Input: part model. Units: mm. Frame: model coordinates. Face numbers are marked on the shaded views. A direction names the side the tool comes from. Give positions to 0.01 mm unless a question says otherwise; leave off trailing zeros. Loops run counter-clockwise (first coordinate to the right, second up) from the corner with the lowest first, then second, coordinate; pieces in that order, holes last. Notation, with made-up numbers: M 76,84 L 116,84 A30 cw 116,123 Z; hole C 46.25,1 d9. An arc over 180 degrees is marked long. Return JSON: item names as keys, results as strings. Group by question number.
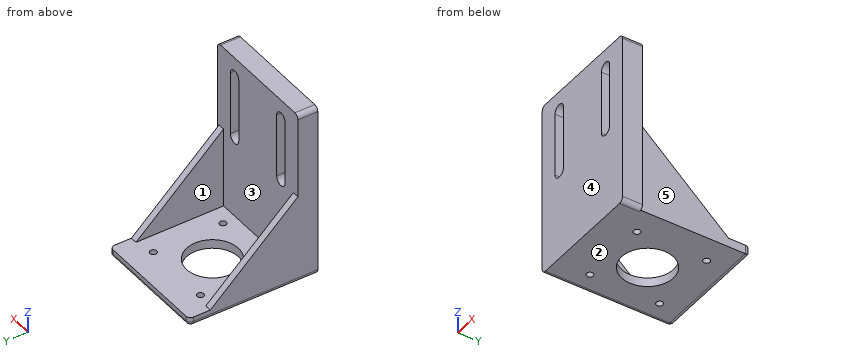
```python
from build123d import *

# Parameters (mm, degrees)
SKETCH1_W               = 53
SKETCH1_H               = 78
BOSS_EXTRUDE1_DEPTH     = 8.85
FILLET2_R               = 2
CUT_EXTRUDE1_DEPTH      = 69.980595097
CUT_EXTRUDE1_DEPTH_BACK = 69.980595097
BOSS_EXTRUDE2_DEPTH     = 48.5
FILLET4_R               = 2
RIB7_REACH              = 96.942
SKETCH4_WALL_W          = 244.959830248
SKETCH4_WALL_H          = 3
RIB8_REACH              = 96.388
SKETCH6_WALL_W          = 243.850654762
SKETCH6_WALL_H          = 3
SKETCH7_R               = 11.5
SKETCH7_R_2             = 1.5
CUT_EXTRUDE2_DEPTH      = 103.611025236


with BuildPart() as part:
    # Sketch1 → Boss-Extrude1 (new body)
    with BuildSketch(Plane(origin=(0, 0, 0), x_dir=(1, 0, 0), z_dir=(0, 1, 0))):
        with Locations((-15.5, -15)):
            Rectangle(SKETCH1_W, SKETCH1_H)
    extrude(amount=BOSS_EXTRUDE1_DEPTH)

    # Fillet2
    fillet2_edges = [part.edges().sort_by_distance(p)[0] for p in [
        (-42, 4.425, -24),
        (11, 4.425, -24),
        (11, 4.425, 54),
        (-42, 4.425, 54),
    ]]
    fillet(fillet2_edges, radius=FILLET2_R)

    # Sketch2 → Cut-Extrude1 (cut, two sides)
    with BuildSketch(Plane(origin=(0, 8.85, 0), x_dir=(1, 0, 0), z_dir=(0, 1, 0))) as cut_extrude1_sk:
        with BuildLine():
            Line((-33.5, -16.75), (-33.5, -45.25))
            ThreePointArc((-33.5, -45.25), (-30.749999997, -48), (-28, -45.249999994))
            Line((-28, -45.249999994), (-28, -16.75))
            ThreePointArc((-28, -16.75), (-30.75, -14), (-33.5, -16.75))
        make_face()
        with BuildLine():
            Line((2.5, -16.75), (2.5, -45.25))
            ThreePointArc((2.5, -45.25), (-0.250000003, -48), (-3, -45.249999994))
            Line((-3, -45.249999994), (-3, -16.75))
            ThreePointArc((-3, -16.75), (-0.25, -14), (2.5, -16.75))
        make_face()
    extrude(amount=CUT_EXTRUDE1_DEPTH, mode=Mode.SUBTRACT)
    extrude(cut_extrude1_sk.sketch, amount=-CUT_EXTRUDE1_DEPTH_BACK, mode=Mode.SUBTRACT)

    # Sketch3 → Boss-Extrude2 (add)
    with BuildSketch(Plane(origin=(0, 8.85, 0), x_dir=(1, 0, 0), z_dir=(0, 1, 0))):
        with BuildLine():
            Line((-42, 20), (10, 20))
            Line((10, 20), (10, 24))
            Line((10, 24), (-40, 24))
            ThreePointArc((-40, 24), (-41.414213562, 23.414213562), (-42, 22))
            Line((-42, 22), (-42, 20))
        make_face()
    extrude(amount=BOSS_EXTRUDE2_DEPTH)

    # Fillet4
    fillet4_edges = [part.edges().sort_by_distance(p)[0] for p in [
        (-42, 57.35, -21),
        (10, 57.35, -22),
        (-15, 57.35, -24),
        (-41.414213562, 57.35, -23.414213562),
    ]]
    fillet(fillet4_edges, radius=FILLET4_R)

    # Sketch4 wall → Rib7 (add, up to next)
    with BuildSketch(Plane(origin=(-42, 28.35, -2), x_dir=(0, 0.734803444627, -0.678280102733), z_dir=(0, -0.678280102733, -0.734803444627)), mode=Mode.PRIVATE) as rib7_sk1:
        with Locations((0, 1.5)):
            Rectangle(SKETCH4_WALL_W, SKETCH4_WALL_H)
    rib7_tool1 = extrude(rib7_sk1.sketch, amount=RIB7_REACH, mode=Mode.PRIVATE) - part.part
    add(rib7_tool1.solids().sort_by_distance((-42, 28.35, -2))[0])

    # Sketch6 wall → Rib8 (add, up to next)
    with BuildSketch(Plane(origin=(10, 28.35, -2), x_dir=(0, -0.734803444627, 0.678280102733), z_dir=(0, -0.678280102733, -0.734803444627)), mode=Mode.PRIVATE) as rib8_sk1:
        with Locations((0, 1.5)):
            Rectangle(SKETCH6_WALL_W, SKETCH6_WALL_H)
    rib8_tool1 = extrude(rib8_sk1.sketch, amount=RIB8_REACH, mode=Mode.PRIVATE) - part.part
    add(rib8_tool1.solids().sort_by_distance((10, 28.35, -2))[0])

    # Sketch7 → Cut-Extrude2 (cut, through all)
    with BuildSketch(Plane.XY.offset(-20)):
        with Locations((-17, 30)):
            Circle(SKETCH7_R)
        with Locations((-32.5, 45.85)):
            Circle(SKETCH7_R_2)
        with Locations((-32.5, 14.85)):
            Circle(SKETCH7_R_2)
        with Locations(Location((-1.5, 14.85, 0), (0, 0, 180))):
            Circle(SKETCH7_R_2)
        with Locations(Location((-1.5, 45.85, 0), (0, 0, 180))):
            Circle(SKETCH7_R_2)
    extrude(amount=-CUT_EXTRUDE2_DEPTH, mode=Mode.SUBTRACT)


solid = part.part
```
Item 1: Pull-direction query (X, two-part tool) for the marked faces 3, 4 and 5; classes: pulls with the +X half, pulls with the -X half, needs draft (parallel to the pull), parting line crosses it, or undercut.
Item 2: Material intervals for line 1 (Y direction, x = -32.5, z = -22.5); line 2 (X direction, y = 11.5, z = 7.5); line 3 (Y direction, x = -1, z = -21), sorted ascending. Write a range as from..to.
Item 3: Section A-A, the plane z = 43.5. Return loops of the section in (x, y), then the cut area to 3 significant figures.
Item 4: Section C-C, the plane y = 14.85. Return loops of the section in (x, z).
Item 5: Section D-D, the plane x = -32.5. Return loops of the section in (y, z), then the cut area to 3 significant figures.
Item 6: Section B-B, the plane x = -17. Return loops of the section in (y, z).
Item 7: Reachability of the marked faces 1 and 2 from +Z, -Z, +X, -X, +Y, -Y: full face, straight path, thin tool, end or side. Return the list, or none.
Item 8: First-contact query: pin 1 Ø4 at (x, y) = (-1.5, 45.85) entering from +Z; pin 2 Ø11 at (y, z) = (29.5, 6.5) entering from -X (3 decimals); pin 3 Ø5 at (y, z) = (14.5, -9.5) entering from +X; pin 4 Ø6 at (x, z) = (3, 10.5) entering from +Y. Flat tips, straight axial feed; report the tip coordinate or a pass-through.
Answer below:
{
 "1": {"face 3": "undercut", "face 4": "needs draft", "face 5": "pulls with the +X half"},
 "2": {"line 1": "0..13.35, 16.35..44.35, 47.35..57.29", "line 2": "-42..-39, 7..10", "line 3": "0..13.44, 16.26..44.44, 47.26..57.35"},
 "3": {"outline": "M -42,0 L -33.5,0 L -33.5,8.85 L -42,8.85 Z; M -28,0 L -3,0 L -3,8.85 L -28,8.85 Z; M 2.5,0 L 11,0 L 11,8.85 L 2.5,8.85 Z", "area": "372 mm^2"},
 "4": {"outline": "M -42,-22 A2 ccw -40,-24 L -34,-24 L -34,-20 L -39,-20 L -39,10.46 L -42,10.46 Z; M -31,-24 L -3,-24 L -3,-20 L -31,-20 Z; M 0,-24 L 10,-24 L 10,10.46 L 7,10.46 L 7,-20 L 0,-20 Z"},
 "5": {"outline": "M 0,-24 L 13.35,-24 L 13.35,-20 L 8.85,-20 L 8.85,14.63 L 0,14.63 Z; M 0,47.37 L 8.85,47.37 L 8.85,54 L 0,54 Z; M 16.35,-24 L 44.35,-24 L 44.35,-20 L 16.35,-20 Z; M 47.35,-24 L 55.35,-24 A2 ccw 57.35,-22 L 57.35,-20 L 47.35,-20 Z", "area": "570 mm^2"},
 "6": {"outline": "M 0,-24 L 18.5,-24 L 18.5,-20 L 8.85,-20 L 8.85,54 L 0,54 Z; M 41.5,-24 L 55.35,-24 A2 ccw 57.35,-22 L 57.35,-20 L 41.5,-20 Z"},
 "7": {"face 1": "+Z, +Y", "face 2": "-Z, +X, -X, +Y, -Y"},
 "8": {"pin 1": "z = -20", "pin 2": "through", "pin 3": "x = 10", "pin 4": "y = 8.85"}
}
